Design review of the part shown in the three views and the two pictorial views. Dimensions are in mm from the part's minimum x, y and z. A direction names the side the tool comes from. Give positions to 0.01 mm unless a question says otherwise; leave off trailing zeros. Write each loop counter-clockwise with the first axis right and the second up, starting at its lowest first coordinate (ties: lowest second). Pieces come first, ordered by that corner, then holes.
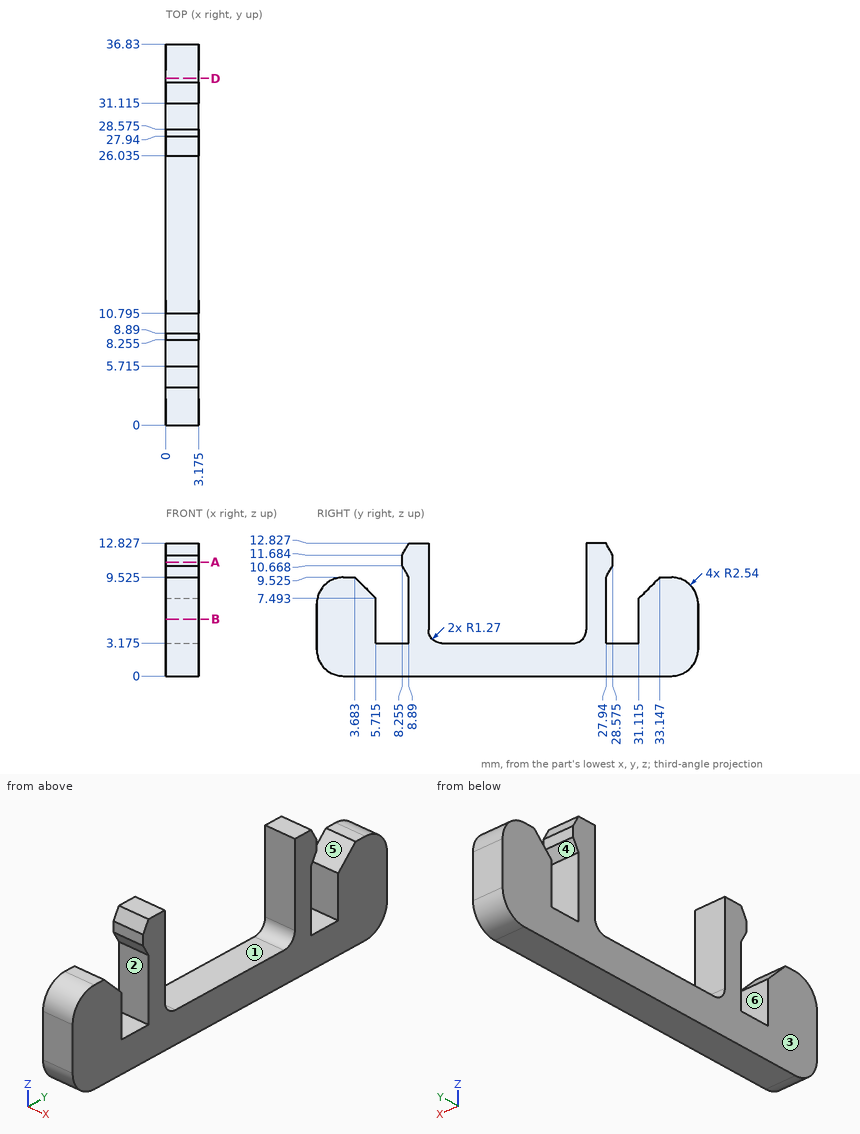
(1) To check wall thickness, follow L1, parallel to Y at x = 0.2, z = 6 (3 decimals); L2, parallel to Y at x = 2.95, z = 11 (3 decimals); L3, parallel to Z at x = 1.85, y = 21 (3 decimals). State the ranges of each line that lie inside material, in increasing order.
Resolved:
L1: y = 0 to 5.715, 8.89 to 10.795, 26.035 to 27.94, 31.115 to 36.83
L2: y = 8.255 to 10.795, 26.035 to 28.575
L3: z = 0 to 3.175
(2) Clearance check with flat-ended pins moving along their axes: P1, Ø1, axis at x = 1.5, y = 18.5, coming from the +Z side (3 decimals); P2, Ø0.6, axis at x = 2, y = 34, coming from the +Z side (3 decimals); P3, Ø1.6, axis at x = 2, z = 8.5, coming from the -Y side. State where each tip first meets the part, or that it passes through.
Resolved:
P1: stops at z = 3.175
P2: stops at z = 9.525
P3: stops at y = 0.1
(3) Consider section D-D, the plane y = 33.5. Give the boundary of the cut face in (x, z) (3 decimals), then the cut area to 3 significant figures.
Resolved:
outline: (0, 0) - (3.175, 0) - (3.175, 9.525) - (0, 9.525) - close
area: 30.2 mm2
(4) Mouldability with a two-part tool opening along Z and no side actions: class the marked faces 4, 5 and 6 as pulls with the +Z half, pulls with the -Z half, needs draft (parallel to the pull), parting line crosses it, or undercut.
Resolved:
face 4: undercut
face 5: pulls with the +Z half
face 6: needs draft
(5) Consider section B-B, the plane z = 5.5. Give the boundary of the cut face in (x, y) (3 decimals), then the cut area to 3 significant figures.
Resolved:
outline: (0, 0) - (3.175, 0) - (3.175, 5.715) - (0, 5.715) - close; (0, 8.89) - (3.175, 8.89) - (3.175, 10.795) - (0, 10.795) - close; (0, 26.035) - (3.175, 26.035) - (3.175, 27.94) - (0, 27.94) - close; (0, 31.115) - (3.175, 31.115) - (3.175, 36.83) - (0, 36.83) - close
area: 48.4 mm2
(6) Tool access review of the marked faces 1, 2 and 3: name each direction out of +Z, -Z, +X, -X, +Y, -Y from which nothing blocks a thin tool from reaching the whole face with its end or side.
Resolved:
face 1: +Z, +X, -X
face 2: +X, -X
face 3: +Z, -Z, -X, +Y, -Y
(7) Consider section A-A, the plane z = 11. Give the boundary of the cut face in (x, y) (3 decimals).
Resolved:
outline: (0, 8.255) - (3.175, 8.255) - (3.175, 10.795) - (0, 10.795) - close; (0, 26.035) - (3.175, 26.035) - (3.175, 28.575) - (0, 28.575) - close
